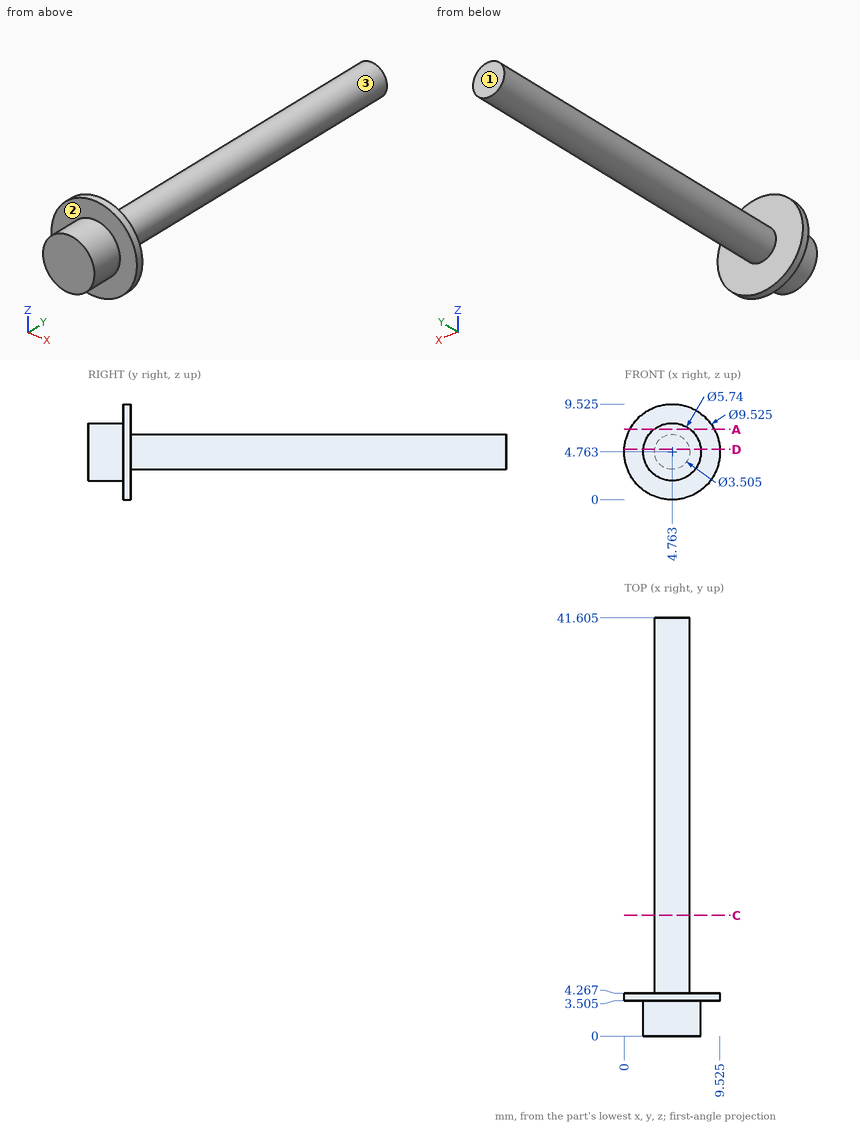
Check sheet for the drawn part. Datum: minimum x, y, z corner. Units: mm. A direction names the side the tool comes from. Round coordinates to 2 decimals unless told otherwise and drop trailing zeros. Loops run counter-clockwise (first coordinate to the right, second up) from the corner with the lowest first, then second, coordinate; pieces in that order, holes last. Notation, with made-up numbers: (-27.75, -29.5) - (-13.75, -29.5) arc R13 cw to (-13.75, -16.5) - close; hole circle Ø11 at (39, 2.5). An arc over 180 degrees is marked (long way). Write item = value, one per line. Start each with the question number.
1. Set-up check for the marked faces 1, 2 and 3: record each of +Z, -Z, +X, -X, +Y, -Y from which the full face is reachable in a straight line by a thin tool's end or side.
2. Section check D-D on z = 5. Enter the section's corners in (x, y) (1 decimal), then the cut area to 3 significant figures.
3. Depth check by flat-ended pin: pin 1 (5 mm diameter, centred on x = 5, y = 29, fed in from +Z) (1 decimal); pin 2 (2 mm diameter, centred on x = 5, z = 7, fed in from +Y) (1 decimal); pin 3 (3 mm diameter, centred on y = 5.5, z = 1.5, fed in from -X) (1 decimal); pin 4 (4 mm diameter, centred on x = 6.5, y = 34, fed in from -Z). Enter the tip coordinate at first touch or a pass-through.
4. Section check C-C on y = 12. Enter the section's corners in (x, z) (1 decimal).
5. Section check A-A on z = 7. Enter the section's corners in (x, y) (1 decimal).
6. Thickness scan on line 1 (Y direction, x = 7.25, z = 2) (1 decimal); line 2 (Y direction, x = 4, z = 2.25); line 3 (Z direction, x = 4.75, y = 40) (1 decimal). Record the ranges inside material, lowest first.
Working result:
q1.face_1 = +Z, -Z, +X, -X, +Y
q1.face_2 = -Y
q1.face_3 = +Y
q2.outline = (0, 3.5) - (1.9, 3.5) - (1.9, 0) - (7.6, 0) - (7.6, 3.5) - (9.5, 3.5) - (9.5, 4.3) - (6.5, 4.3) - (6.5, 41.6) - (3, 41.6) - (3, 4.3) - (0, 4.3) - close
q2.area = 157 mm^2
q3.pin_1 = 6.5
q3.pin_2 = 41.6
q3.pin_3 = 0.7
q3.pin_4 = 3.01
q4.outline = circle Ø3.5 at (4.8, 4.8)
q5.outline = (0.6, 3.5) - (3, 3.5) - (3, 0) - (6.6, 0) - (6.6, 3.5) - (9, 3.5) - (9, 4.3) - (0.6, 4.3) - close
q6.line_1 = 3.5 to 4.3
q6.line_2 = 0 to 4.27
q6.line_3 = 3 to 6.5
